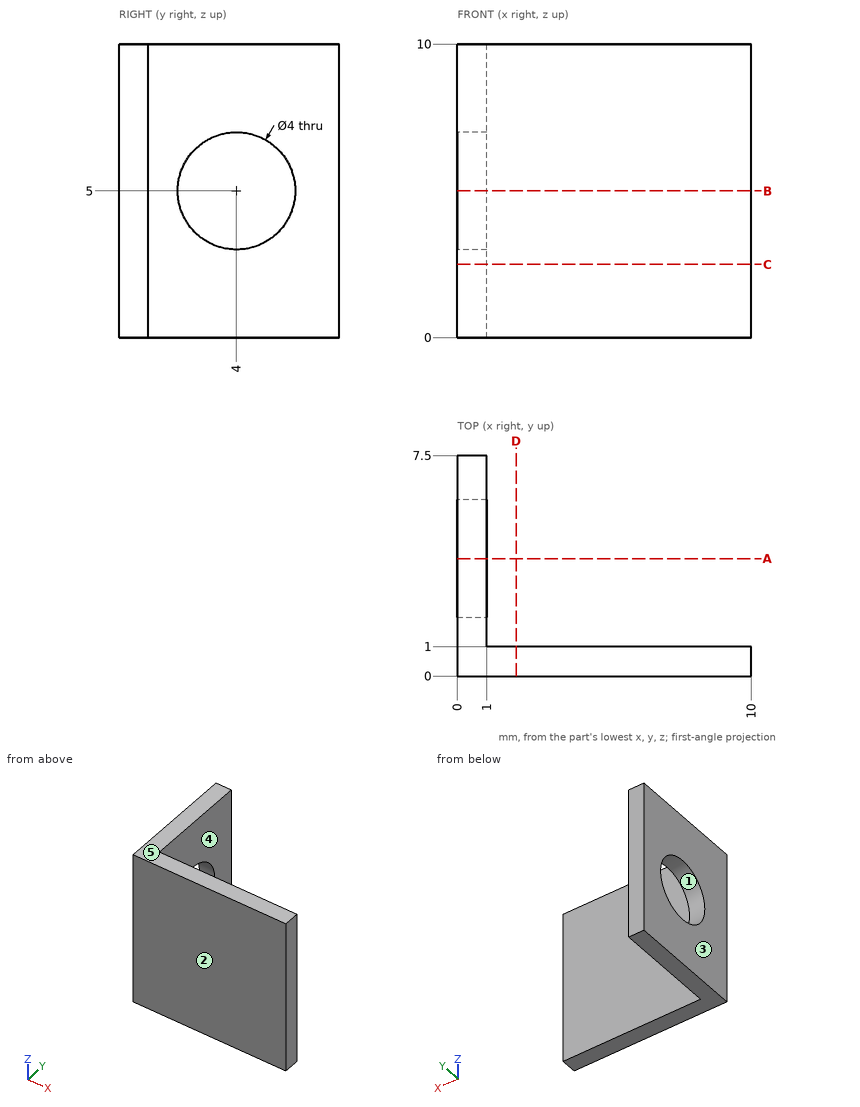
For this review, use the dimensioned drawing (mm, ordinates from the lowest corner) and the shaded views. A direction names the side the tool comes from. Give positions to 0.01 mm unless a question says otherwise; leave off trailing zeros. Order: outer loops, then holes, each group sorted by start corner. A loop starts at its lowest first (then second) coordinate and runs counter-clockwise, first axis right, second up. Notation, with made-up numbers: (-34, -22.75) - (18, -22.75) arc R18 cw to (18, 8.25) - close; hole circle Ø6 at (1.25, 64.25). An arc over 180 degrees is marked (long way). Use a Markdown table: item, result. Add a question column.
(1) Add section D-D on x = 2. Give the boundary of the cut face in (y, z).
(2) Machinability: for the marked faces 4 and 5, which of the approach directions +Z, -Z, +X, -X, +Y, -Y give a long, thin tool a straight path to every point of the face, cutting with its end or side? Answer none if there is none.
(3) Wall thickness on probe 1 along Z at (x, y) = (0.55, 4); probe 2 along Y at (x, z) = (3, 3): over which ranges is each line inside the solid? List them lowest first. Write a range as [from, to].
(4) Clearance check with flat-ended pins moving along their axes: P1, Ø2.5, axis at x = 3.5, z = 5.5, coming from the +Y side; P2, Ø2, axis at y = 4.5, z = 5, coming from the +X side; P3, Ø1.5, axis at y = 3, z = 8, coming from the +X side. State where each tip first meets the part, or that it passes through.
(5) Add section B-B on z = 5. Give the boundary of the cut face in (x, y).
(6) Add section A-A on y = 4. Give the boundary of the cut face in (x, z).
(7) Mouldability with a two-part tool opening along Y and no side actions: class the marked faces 1, 2 and 3 as +Y half, -Y half, draft (parallel to the pull), parting line (faces both ways), or undercut.
(8) Add section C-C on z = 2.5. Give the boundary of the cut face in (x, y).
Report:
| question | item | result |
|---|---|---|
| 1 | outline | (0, 0) - (1, 0) - (1, 10) - (0, 10) - close |
| 2 | face 4 | +Z, -Z, +X, +Y |
| 2 | face 5 | +Z, +X, -X, +Y, -Y |
| 3 | probe 1 | z = [0, 3], [7, 10] |
| 3 | probe 2 | y = [0, 1] |
| 4 | P1 | stops at y = 1 |
| 4 | P2 | passes through |
| 4 | P3 | stops at x = 1 |
| 5 | outline | (0, 0) - (10, 0) - (10, 1) - (1, 1) - (1, 2) - (0, 2) - close; (0, 6) - (1, 6) - (1, 7.5) - (0, 7.5) - close |
| 6 | outline | (0, 0) - (1, 0) - (1, 3) - (0, 3) - close; (0, 7) - (1, 7) - (1, 10) - (0, 10) - close |
| 7 | face 1 | undercut |
| 7 | face 2 | -Y half |
| 7 | face 3 | draft |
| 8 | outline | (0, 0) - (10, 0) - (10, 1) - (1, 1) - (1, 7.5) - (0, 7.5) - close |
